Can you work these out from the model? Positions are in its coordinate system, mm. A direction names the side the tool comes from. Round coordinates to 2 decimals unless told otherwise and drop trailing zeros. Write each loop counter-clockwise with the first axis right and the second up, starting at its lowest first coordinate (ties: lowest second). Pieces come first, ordered by that corner, then holes.
Q1. I'm going to push flat-ended pins straight in: pin 1 Ø1.8 at (x, y) = (120.5, 4.5) entering from +Z; pin 2 Ø1.8 at (x, y) = (163.5, 4.5) entering from +Z; pin 3 Ø6 at (x, y) = (101.5, 1.5) entering from -Z; pin 4 Ø2 at (y, z) = (5, 5.5) entering from -X. Where does each tip first touch, or does it pass through?
Q2. If we section it at B-B (x = 153): Please give me the cut outline in (y, z), plus the area to 3 significant figures.
Q3. If we section it at A-A (x = 54.5): Please give me the cut outline in (y, z), plus the area to 3 significant figures.
Q4. Please list where these lines run through material, in increasing order: line 1 along Z through (x, y) = (54.5, 4.75); line 2 along Y through (x, z) = (5, 0.5); line 3 along Y through (x, z) = (7, 4).
Q5. For faces 1 (the flat face through (90, 10, 5)), 2 (the flat face through (7.57, 3.55, 3.4)), which set-ups out of +Z, -Z, +X, -X, +Y, -Y let a thin tool reach every point of the face, with its end or its side?
Q6. If we section it at C-C (x = 15): Please give me the cut outline in (y, z).
Q7. We'd pull the mould along X, two halves only. Please class faces 3 (the flat face through (153, 2.05, 7)), 4 (the flat face through (157, 5, 7)), 5 (the flat face through (87, 5, 0)): +X half, -X half, draft (parallel to the pull), parting line (faces both ways), or undercut.
Autodesk Inventor part; units mm, degrees
ref_plane "YZ Plane" through (0, 0, 0) normal (1, 0, 0) x (0, 1, 0)
ref_plane "XZ Plane" through (0, 0, 0) normal (0, 1, 0) x (-1, 0, 0)
ref_plane "XY Plane" through (0, 0, 0) normal (0, 0, 1) x (1, 0, 0)
sketch "Sketch1" plane through (0, 0, 0) normal (0, 0, 1) x (1, 0, 0)
  line L0 (0, 0) -> (177, 0)
  line L1 (177, 0) -> (177, 10)
  line L2 (177, 10) -> (0, 10)
  line L3 (0, 10) -> (0, 0)
  circle A0 centre (59.5, 5) radius 1.6
  circle A1 centre (119.5, 5) radius 1.6
  circle A2 centre (162, 5) radius 1.6
  circle A3 centre (153, 5) radius 1.6
  circle A4 centre (15, 5) radius 1.6
  circle A5 centre (5, 5) radius 1.6
  dimension "d1" = 10
  dimension "d2" = 90
  dimension "d4" = 3.2
  dimension "d6" = 3.2
  dimension "d7" = 3.2
  dimension "d8" = 60
  dimension "d9" = 42.5
  dimension "d26" = 3.2
  dimension "d27" = 33.5
  dimension "d28" = 3.2
  dimension "d29" = 44.5
  dimension "d32" = 15
  dimension "d33" = 15
  dimension "d61" = 3.2
  dimension "d62" = 10
  dimension "d63" = 9
ref_plane "Work Plane2" through (0, 0, 0) normal (0, -1, 0) x (1, 0, 0)
sketch "Sketch2" plane through (0, 0, 0) normal (0, -1, 0) x (1, 0, 0)
  circle A0 centre (54.5, 7) radius 1.6
  circle A1 centre (137.5, 7) radius 1.6
  circle A2 centre (96, 7) radius 1.6
  point P0 (0, 0)
  dimension "d13" = 3.2
  dimension "d15" = 3.2
  dimension "d16" = 83
  dimension "d17" = 3.2
  dimension "d18" = 41.5
  dimension "d64" = 54.5
  dimension "d65" = 41.5
ref_plane "Work Plane1" through (0, 0, 11) normal (0, 0, 1) x (1, 0, 0)
extrude "klocek" add sketch "Sketch1" along normal blind 11
ref_plane "Work Plane3" through (0, 0, 0) normal (0, -1, 0) x (1, 0, 0)
extrude "prowadzenie osi" cut sketch "Sketch2" against normal up to next
ref_plane "Work Plane4" through (0, 0, 0) normal (0, -1, 0) x (1, 0, 0)
sketch "Sketch7" plane through (0, 0, 0) normal (0, -1, 0) x (1, 0, 0)
  line L0 (0, 11) -> (0, 3)
  line L1 (0, 11) -> (177, 11)
  line L2 (0, 11) -> (38, 11)
  line L3 (38, 11) -> (0, 3)
  point P0 (0, -1.8333)
  dimension "d86" = 8
  dimension "d87" = 38
sketch "Sketch8" plane through (0, 0, 0) normal (0, -1, 0) x (1, 0, 0)
  line L0 (177, 0) -> (177, 11)
  line L1 (177, 11) -> (177, 3)
  line L2 (177, 11) -> (0, 11)
  line L3 (177, 11) -> (137, 11)
  line L4 (137, 11) -> (177, 3)
  point P0 (0, 0)
  point P1 (40.8333, 11)
  dimension "d80" = 8
  dimension "d81" = 40
extrude "przedni skos" cut sketch "Sketch7" against normal up to next
extrude "tylni skos" cut sketch "Sketch8" against normal up to next
ref_plane "Work Plane7" through (0, 0, 11) normal (0, 0, 1) x (1, 0, 0)
sketch "Sketch5" plane through (0, 0, 11) normal (0, 0, 1) x (1, 0, 0)
  line L0 (62.9064, 5) -> (61.2032, 2.05)
  line L1 (61.2032, 2.05) -> (57.7968, 2.05)
  line L2 (57.7968, 2.05) -> (56.0936, 5)
  line L3 (56.0936, 5) -> (57.7968, 7.95)
  line L4 (57.7968, 7.95) -> (61.2032, 7.95)
  line L5 (61.2032, 7.95) -> (62.9064, 5)
  line L6 (122.9064, 5) -> (121.2032, 2.05)
  line L7 (121.2032, 2.05) -> (117.7968, 2.05)
  line L8 (117.7968, 2.05) -> (116.0936, 5)
  line L9 (116.0936, 5) -> (117.7968, 7.95)
  line L10 (117.7968, 7.95) -> (121.2032, 7.95)
  line L11 (121.2032, 7.95) -> (122.9064, 5)
  point P0 (59.5, 5)
  point P1 (119.5, 5)
  point P2 (119.5, 5)
  dimension "d44" = 5.9
  dimension "d45" = 5.9
extrude "hex insert middle" cut sketch "Sketch5" against normal blind 3
ref_plane "Work Plane6" through (0, 0, 11) normal (0, 0, 1) x (1, 0, 0)
sketch "Sketch9" plane through (0, 0, 11) normal (0, 0, 1) x (1, 0, 0)
  line L0 (156.4064, 5) -> (154.7032, 2.05)
  line L1 (154.7032, 2.05) -> (151.2968, 2.05)
  line L2 (151.2968, 2.05) -> (149.5936, 5)
  line L3 (149.5936, 5) -> (151.2968, 7.95)
  line L4 (151.2968, 7.95) -> (154.7032, 7.95)
  line L5 (154.7032, 7.95) -> (156.4064, 5)
  point P0 (0, 0)
  point P1 (153, 5)
  point P2 (153, 5)
  dimension "d51" = 5.9
extrude "hex insert rear 1" cut sketch "Sketch9" against normal blind 6
ref_plane "Work Plane5" through (0, 0, 11) normal (0, 0, 1) x (1, 0, 0)
sketch "Sketch10" plane through (0, 0, 11) normal (0, 0, 1) x (1, 0, 0)
  line L0 (160.2968, 7.95) -> (163.7032, 7.95)
  line L1 (163.7032, 7.95) -> (165.4064, 5)
  line L2 (165.4064, 5) -> (163.7032, 2.05)
  line L3 (163.7032, 2.05) -> (160.2968, 2.05)
  line L4 (160.2968, 2.05) -> (158.5936, 5)
  line L5 (158.5936, 5) -> (160.2968, 7.95)
  point P0 (0, 0)
  point P1 (162, 5)
  point P2 (162, 5)
  dimension "d72" = 5.9
extrude "hex insert rear 2" cut sketch "Sketch10" against normal blind 7.5
sketch "Sketch13" plane through (0, 0, 11) normal (0, 0, 1) x (1, 0, 0)
  circle A0 centre (5, 5) radius 1.6
  line L0 (8.4064, 5) -> (6.7032, 2.05)
  line L1 (6.7032, 2.05) -> (3.2968, 2.05)
  line L2 (3.2968, 2.05) -> (1.5936, 5)
  line L3 (1.5936, 5) -> (3.2968, 7.95)
  line L4 (3.2968, 7.95) -> (6.7032, 7.95)
  line L5 (6.7032, 7.95) -> (8.4064, 5)
  point P0 (0, 0)
  dimension "d90" = 5.9
extrude "Extrusion18" cut sketch "Sketch13" against normal blind 9
sketch "Sketch16" plane through (0, 0, 11) normal (0, 0, 1) x (1, 0, 0)
  circle A0 centre (15, 5) radius 1.6
  line L0 (18.4064, 5) -> (16.7032, 2.05)
  line L1 (16.7032, 2.05) -> (13.2968, 2.05)
  line L2 (13.2968, 2.05) -> (11.5936, 5)
  line L3 (11.5936, 5) -> (13.2968, 7.95)
  line L4 (13.2968, 7.95) -> (16.7032, 7.95)
  line L5 (16.7032, 7.95) -> (18.4064, 5)
  point P0 (0, 0)
  dimension "d93" = 5.9
extrude "Extrusion19" cut sketch "Sketch16" against normal blind 7.5
properties part number "wheel_support_long"
A:
1. pin 1: stops at z = 8
1. pin 2: stops at z = 3.5
1. pin 3: stops at z = 0
1. pin 4: stops at x = 8.06
2. outline: (0, 0) - (3.4, 0) - (3.4, 5) - (2.05, 5) - (2.05, 7.8) - (0, 7.8) - close; (6.6, 0) - (10, 0) - (10, 7.8) - (7.95, 7.8) - (7.95, 5) - (6.6, 5) - close
2. area: 45.5 mm2
3. outline: (0, 0) - (10, 0) - (10, 5.4) - (0, 5.4) - close; (0, 8.6) - (10, 8.6) - (10, 11) - (0, 11) - close
3. area: 78.0 mm2
4. line 1: z = 0 to 5.4, 8.6 to 11
4. line 2: y = 0 to 3.4, 6.6 to 10
4. line 3: y = 0 to 2.56, 7.44 to 10
5. face 1: +Z, -Z, +X, -X, +Y
5. face 2: +Z
6. outline: (0, 0) - (3.4, 0) - (3.4, 3.5) - (2.05, 3.5) - (2.05, 6.16) - (0, 6.16) - close; (6.6, 0) - (10, 0) - (10, 6.16) - (7.95, 6.16) - (7.95, 3.5) - (6.6, 3.5) - close
7. face 3: undercut
7. face 4: +X half
7. face 5: draft
